Work out the finished part from the listing and answer in its coordinate system (mm). A direction names the side the tool comes from. Coordinates: 2 decimals unless noted, no trailing zeros. Order: outer loops, then holes, each group sorted by start corner. A loop starts at its lowest first (then second) coordinate and runs counter-clockwise, first axis right, second up. Notation, with made-up numbers: (7.5, 9.5) - (32.5, 9.5) arc R17 ccw to (32.5, 24.5) - close; hole circle Ø4 at (60, -11). An arc over 180 degrees is marked (long way). Answer as a JSON object with one key per item and string values. Group by question number.
1) Section C-C (x = -48) is taken. Give the vertices of the cut face in (y, z), plus the area to 3 significant figures.
2) Section B-B (y = 12.5) is taken. Give the vertices of the cut face in (x, z), plus the area to 3 significant figures.
3) The mould has two halves that part along X. Classify faces 3 (the face through (-158.437, -2, 12)), 4 (the face through (-110.11, -7.32, 12.32)), 5 (the face through (-78, 25, 12)): released by +X, released by -X, zero draft, split by the parting line, or undercut.
4) Section D-D (y = 23) is taken. Give the vertices of the cut face in (x, z), plus the area to 3 significant figures.
5) Find the intervals of material crossed by line 1 along X through (y, z) = (11.5, 9); line 2 along Y through (x, z) = (34, 22.5); line 3 along Y through (x, z) = (-143.5, 22), in increasing order.
6) A tool of negligible diameter and unlimited length cuts with its end or side. For faces 1 (the face through (-119, 0, 12)), 2 (the face through (-22, 9, 0)), from which of +Z, -Z, +X, -X, +Y, -Y can it reach the whole face along a straight path? Write none if from no direction.
7) Section A-A (z = 22.75) is taken. Give the vertices of the cut face in (x, y) (1 decimal).
8) Each of these flat-tipped pins is pushed along its axis until it touches: P1, Ø7.5, axis at x = -144.5, z = 8.5, coming from the -Y side; P2, Ø4, axis at y = 18, z = 11, coming from the +X side; P3, Ø1, axis at x = 11, z = 18, coming from the -Y side. Where does it stop, or does it pass through?
from build123d import *

# Parameters (mm, degrees)
F0_R     = 17.5
F0_W     = 8
F0_H     = 15
F0_W_2   = 10
F0_H_2   = 30
F1_DEPTH = 25


with BuildPart() as f1:
    # F0 (on Top) → F1 (new body)
    with BuildSketch(Plane.XY):
        Polygon((-100.000008, 0), (0, 0), (0, 25), (-158.437499, 25), (-158.437499, 0), (-148.437499, 0), (-133.125003, 0), (-125.125003, 0), (-112.812507, 0), align=None)
        with BuildLine():
            Line((0, 25), (0, 0))
            ThreePointArc((0, 0), (67.691742, 12.5), (0, 25))
        make_face()
        with Locations((32.691742, 12.5)):
            Circle(F0_R, mode=Mode.SUBTRACT)
        Polygon((-107.33281, -14.84021), (-100.000008, 0), (-112.812507, 0), align=None)
        with Locations((-129.125003, -7.5)):
            Rectangle(F0_W, F0_H)
        with Locations((-153.437499, -15)):
            Rectangle(F0_W_2, F0_H_2)
    extrude(amount=F1_DEPTH)


solid = f1.part
Report:
{
 "1": {"outline": "(0, 0) - (25, 0) - (25, 25) - (0, 25) - close", "area": "625 mm²"},
 "2": {"outline": "(-158.44, 0) - (15.19, 0) - (15.19, 25) - (-158.44, 25) - close; (50.19, 0) - (67.69, 0) - (67.69, 25) - (50.19, 25) - close", "area": "4,780 mm²"},
 "3": {"face 3": "released by -X", "face 4": "undercut", "face 5": "zero draft"},
 "4": {"outline": "(-158.44, 0) - (18.69, 0) - (18.69, 25) - (-158.44, 25) - close; (46.69, 0) - (66.08, 0) - (66.08, 25) - (46.69, 25) - close", "area": "4,910 mm²"},
 "5": {"line 1": "x = -158.44 to 15.22, 50.16 to 67.68", "line 2": "y = -22.48 to -4.95, 29.95 to 47.48", "line 3": "y = 0 to 25"},
 "6": {"face 1": "+Z, -Z, -Y", "face 2": "-Z, +X, -X, +Y, -Y"},
 "7": {"outline": "(-158.4, -30) - (-148.4, -30) - (-148.4, 0) - (-133.1, 0) - (-133.1, -15) - (-125.1, -15) - (-125.1, 0) - (-112.8, 0) - (-107.3, -14.8) - (-100, 0) - (0, 0) arc R35 ccw (long way) to (0, 25) - (-158.4, 25) - close; hole circle Ø35 at (32.7, 12.5)"},
 "8": {"P1": "stops at y = 0", "P2": "stops at x = 67.52", "P3": "stops at y = -15.36"}
}
